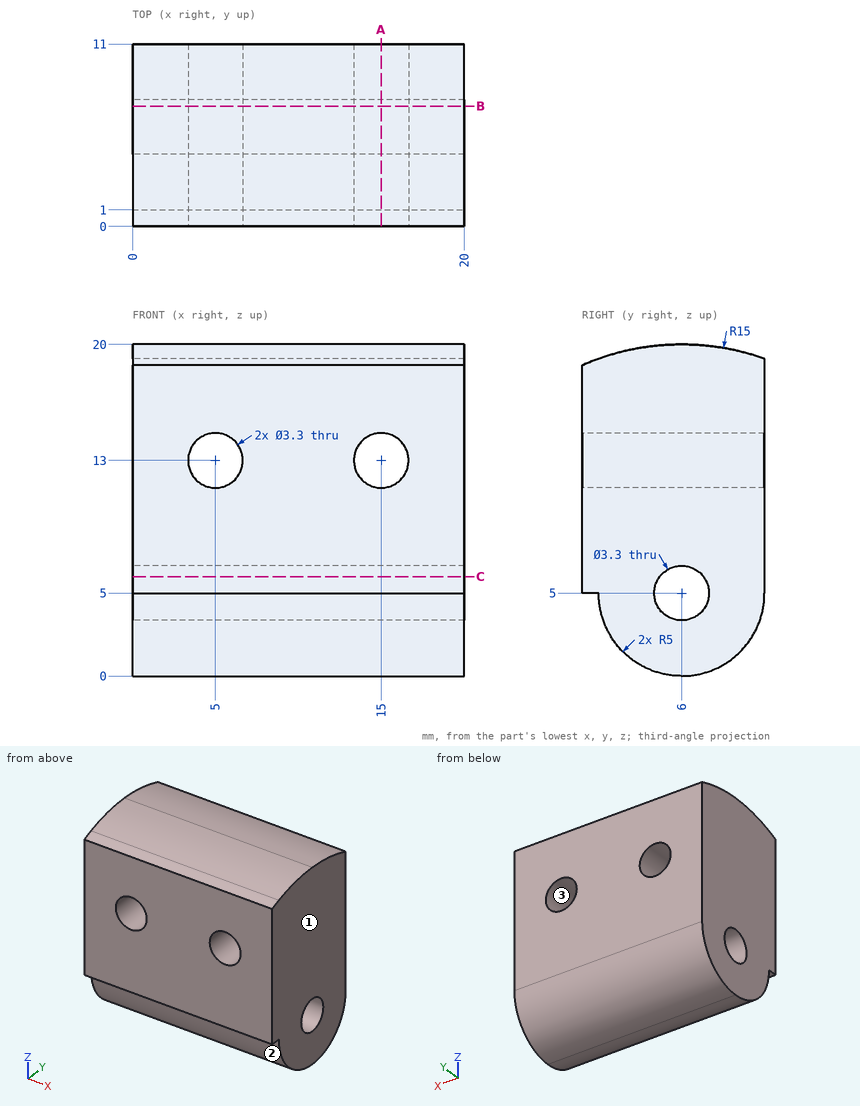
The drawing under review shows one solid part. Ordinate dimensions are in mm from its lowest x, y, z. Give positions to 0.01 mm unless a question says otherwise; leave off trailing zeros. Order: outer loops, then holes, each group sorted by start corner. A loop starts at its lowest first (then second) coordinate and runs counter-clockwise, first axis right, second up. Notation, with made-up numbers: M 12.25,-19 L 60.25,-19 A21 ccw 60.25,-14 Z; hole C 53,-9 d4. An arc over 180 degrees is marked long. Answer in a Markdown table with one row per item. Add a question column.
1. To check wall thickness, follow line 1 along X through (y, z) = (4.5, 13); line 2 along Z through (x, y) = (5.5, 7.5) (1 decimal); line 3 along Z through (x, y) = (15, 7). State the ranges of each line that lie inside material, in increasing order.
2. Add section A-A on x = 15. Count the separate pieces of the cut face and the enclosed holes in it, plus the area to 3 significant figures.
3. Mouldability with a two-part tool opening along X and no side actions: class the marked faces 1, 2 and 3 as released by +X, released by -X, zero draft, split by the parting line, or undercut.
4. Add section B-B on y = 7.25. State the section outline as (x, z) points, plus the area to 3 significant figures.
5. Add section C-C on z = 6. State the section outline as (x, y) points, plus the area to 4 significant figures.
6. For pin 1 Ø2 at (x, y) = (14, 10) entering from -Z; pin 2 Ø2 at (y, z) = (6, 5) entering from -X; pin 3 Ø1.5 at (x, y) = (11.5, 9) entering from -Z (3 decimals); pin 4 Ø2 at (x, y) = (12, 4.5) entering from +Z, all flat-tipped, find the tip position at first contact; note any pin that passes through.
The answers:
| question | item | result |
|---|---|---|
| 1 | line 1 | 0 to 3.35, 6.65 to 13.35, 16.65 to 20 |
| 1 | line 2 | 0.2 to 4.3, 5.7 to 11.4, 14.6 to 19.9 |
| 1 | line 3 | 0.1 to 3.69, 6.31 to 11.35, 14.65 to 19.97 |
| 2 | separate pieces | 2 |
| 2 | enclosed holes | 1 |
| 2 | area | 156 mm2 |
| 3 | face 1 | released by +X |
| 3 | face 2 | zero draft |
| 3 | face 3 | undercut |
| 4 | outline | M 0,0.16 L 20,0.16 L 20,3.92 L 0,3.92 Z; M 0,6.08 L 20,6.08 L 20,19.95 L 0,19.95 Z; hole C 5,13 d3.3; hole C 15,13 d3.3 |
| 4 | area | 336 mm2 |
| 5 | outline | M 0,0 L 20,0 L 20,4.69 L 0,4.69 Z; M 0,7.31 L 20,7.31 L 20,11 L 0,11 Z |
| 5 | area | 167.5 mm2 |
| 6 | pin 1 | z = 1 |
| 6 | pin 2 | through |
| 6 | pin 3 | z = 0.535 |
| 6 | pin 4 | z = 19.99 |
